from build123d import *

# Parameters (mm, degrees)
SZKIC1_W                       = 47
SZKIC1_H                       = 39.6
DODANIE_WYCI_GNI_CIE1_DEPTH    = 75
OTW_R_GWINTOWANY_M4X0_72_D     = 3.3
OTW_R_GWINTOWANY_M4X0_72_DEPTH = 15
OTW_R_GWINTOWANY_M4X0_72_TIP   = 0.991420021
SFAZOWANIE1_SIZE               = 0.5


with BuildPart() as part:
    # Szkic1 → Dodanie-wyciągnięcie1 (new body)
    with BuildSketch(Plane.XY):
        with Locations((23.5, 19.8)):
            Rectangle(SZKIC1_W, SZKIC1_H)
    extrude(amount=DODANIE_WYCI_GNI_CIE1_DEPTH)

    # Otwór gwintowany M4x0.72
    with Locations(Plane.XY.offset(75)):
        with Locations((4.5, 34.8), (23.5, 32.8), (42.5, 34.8), (42.5, 4.8), (23.5, 6.8), (4.5, 4.8)):
            Hole(OTW_R_GWINTOWANY_M4X0_72_D / 2, depth=OTW_R_GWINTOWANY_M4X0_72_DEPTH)
            with Locations((0, 0, -(OTW_R_GWINTOWANY_M4X0_72_DEPTH + OTW_R_GWINTOWANY_M4X0_72_TIP / 2))):  # 118° drill point
                Cone(0, OTW_R_GWINTOWANY_M4X0_72_D / 2, OTW_R_GWINTOWANY_M4X0_72_TIP, mode=Mode.SUBTRACT)

    # Sfazowanie1
    sfazowanie1_edges = [part.edges().sort_by_distance(p)[0] for p in [
        (6.15, 4.8, 75),
        (25.15, 6.8, 75),
        (44.15, 4.8, 75),
        (44.15, 34.8, 75),
        (25.15, 32.8, 75),
        (6.15, 34.8, 75),
    ]]
    chamfer(sfazowanie1_edges, length=SFAZOWANIE1_SIZE)


solid = part.part
Source: CAD feature listing. Evaluate the final solid. Frame: model axes, mm. A direction names the side the tool comes from. Coordinates: 2 decimals unless noted, no trailing zeros. Use a Markdown table: item, result.
1) First-contact query: pin 1 Ø5 at (x, y) = (32, 13) entering from -Z; pin 2 Ø3 at (x, y) = (23.5, 6.8) entering from +Z. Flat tips, straight axial feed; report the tip coordinate or a pass-through.
Conclusion:
| item | result |
|---|---|
| pin 1 | stops at z = 0 |
| pin 2 | stops at z = 59.91 |
2) Mould query, pull axis X, two halves, no side actions, for faces 1 (the conical face through (42.214, 4.813, 59.181)), 2 (the flat face through (47, 20, 37)), 3 (the flat face through (23, 39.6, 37)). Classes: pulls with the +X half, pulls with the -X half, needs draft (parallel to the pull), parting line crosses it, or undercut.
Conclusion:
| item | result |
|---|---|
| face 1 | undercut |
| face 2 | pulls with the +X half |
| face 3 | needs draft |
3) Ray query, L1, parallel to Y at x = 23.5, z = 65.25; L2, parallel to X at y = 34.8, z = 69.5; L3, parallel to Y at x = 42.5, z = 70.25. Return the intervals inside material, ascending.
Conclusion:
| item | result |
|---|---|
| L1 | y = 0 to 5.15, 8.45 to 31.15, 34.45 to 39.6 |
| L2 | x = 0 to 2.85, 6.15 to 40.85, 44.15 to 47 |
| L3 | y = 0 to 3.15, 6.45 to 33.15, 36.45 to 39.6 |
4) Reachability of faces 4 (the flat face through (0, 20, 37)), 5 (the cylindrical face through (25.15, 32.87, 67.15)) from +Z, -Z, +X, -X, +Y, -Y: full face, straight path, thin tool, end or side. Return the list, or none.
Conclusion:
| item | result |
|---|---|
| face 4 | +Z, -Z, -X, +Y, -Y |
| face 5 | +Z |
